Source: CAD feature listing. Evaluate the final solid. Frame: model axes, mm. A direction names the side the tool comes from. Coordinates: 2 decimals unless noted, no trailing zeros. Write each loop counter-clockwise with the first axis right and the second up, starting at its lowest first coordinate (ties: lowest second). Pieces come first, ordered by that corner, then holes. Notation, with made-up numbers: (-11.75, 64.5) - (34.25, 64.5) arc R10 cw to (34.25, 73.5) - close; hole circle Ø6 at (77.5, 89.5). An arc over 180 degrees is marked (long way). One line per item, written item: value.
from build123d import *

# Parameters (mm, degrees)
SALIENTE_EXTRUIR1_DEPTH = 2
CROQUIS2_W              = 12.25
CROQUIS2_H              = 10
SALIENTE_EXTRUIR2_DEPTH = 7
REDONDEO1_R             = 5
CROQUIS3_R              = 0.6
CORTAR_EXTRUIR1_DEPTH   = 7.2
SALIENTE_EXTRUIR3_DEPTH = 1.8
CROQUIS5_W              = 12.25
CROQUIS5_H              = 15.8
SALIENTE_EXTRUIR4_DEPTH = 7
REDONDEO2_R             = 5
CROQUIS6_R              = 0.6
CORTAR_EXTRUIR2_DEPTH   = 9.8
CROQUIS7_W              = 2.8
CROQUIS7_H              = 5.8
SALIENTE_EXTRUIR5_DEPTH = 1.8
CROQUIS8_R              = 1.5
CORTAR_EXTRUIR3_DEPTH   = 13.8
CROQUIS9_R              = 3
CORTAR_EXTRUIR4_DEPTH   = 6
CROQUIS10_R             = 12
SALIENTE_EXTRUIR6_DEPTH = 2
CORTAR_EXTRUIR5_DEPTH   = 2.2
CROQUIS12_R             = 1.6
CORTAR_EXTRUIR6_DEPTH   = 4.2
CROQUIS14_R             = 1.6
SALIENTE_EXTRUIR7_DEPTH = 2


with BuildPart() as part:
    # Croquis1 → Saliente-Extruir1 (new body)
    with BuildSketch(Plane(origin=(0, 0, 45.55), x_dir=(-1, 0, 0), z_dir=(0, 0, -1))):
        with BuildLine():
            Line((-17.240678969, 0.142768675), (-17.240678969, -9.857231325))
            ThreePointArc((-17.240678969, -9.857231325), (-7.189890991, -10.796826624), (2.512589694, -13.583051105))
            ThreePointArc((2.512589694, -13.583051105), (7.914003263, -15.134154499), (13.509321031, -15.657231325))
            Line((13.509321031, -15.657231325), (25.509321031, -15.657231325))
            Line((25.509321031, -15.657231325), (25.509321031, -3.657231325))
            ThreePointArc((25.509321031, -3.657231325), (21.994602405, 4.82805005), (13.509321031, 8.342768675))
            ThreePointArc((13.509321031, 8.342768675), (1.641917085, 6.787620461), (-9.424079639, 2.227195163))
            ThreePointArc((-9.424079639, 2.227195163), (-13.195803851, 0.672823972), (-17.240678969, 0.142768675))
        make_face()
    extrude(amount=SALIENTE_EXTRUIR1_DEPTH)

    # Croquis2 → Saliente-Extruir2 (add)
    with BuildSketch(Plane(origin=(17.240678969, 0, 0), x_dir=(0, 0, -1), z_dir=(1, 0, 0))):
        with Locations((-49.675, -4.857231325)):
            Rectangle(CROQUIS2_W, CROQUIS2_H)
    extrude(amount=SALIENTE_EXTRUIR2_DEPTH)

    # Redondeo1
    redondeo1_edges = [part.edges().sort_by_distance(p)[0] for p in [
        (24.240678969, -9.857231325, 49.675),
    ]]
    fillet(redondeo1_edges, radius=REDONDEO1_R)

    # Croquis3 → Cortar-Extruir1 (cut)
    with BuildSketch(Plane(origin=(0, 0.142768675, 0), x_dir=(1, 0, 0), z_dir=(0, 1, 0))):
        with Locations(Location((20.740678969, -50.8, 0), (0, 0, 270))):
            Circle(CROQUIS3_R)
    extrude(amount=-CORTAR_EXTRUIR1_DEPTH, mode=Mode.SUBTRACT)

    # Croquis4 → Saliente-Extruir3 (add)
    with BuildSketch(Plane.XY.offset(55.8)):
        with BuildLine():
            Line((19.340678969, -1.957231325), (19.340678969, -7.755506674))
            ThreePointArc((19.340678969, -7.755506674), (21.32634433, -6.872175493), (22.140678969, -4.857231325))
            Line((22.140678969, -4.857231325), (22.140678969, -1.957231325))
            Line((22.140678969, -1.957231325), (19.340678969, -1.957231325))
        make_face()
    extrude(amount=SALIENTE_EXTRUIR3_DEPTH)

    # Croquis5 → Saliente-Extruir4 (add)
    with BuildSketch(Plane.ZY.offset(23.759321031)):
        with Locations((49.675, -7.757231325)):
            Rectangle(CROQUIS5_W, CROQUIS5_H)
    extrude(amount=SALIENTE_EXTRUIR4_DEPTH)

    # Redondeo2
    redondeo2_edges = [part.edges().sort_by_distance(p)[0] for p in [
        (-30.759321031, -15.657231325, 49.675),
    ]]
    fillet(redondeo2_edges, radius=REDONDEO2_R)

    # Croquis6 → Cortar-Extruir2 (cut)
    with BuildSketch(Plane(origin=(0, 0.142768675, 0), x_dir=(1, 0, 0), z_dir=(0, 1, 0))):
        with Locations(Location((-27.259321031, -50.8, 0), (0, 0, 270))):
            Circle(CROQUIS6_R)
    extrude(amount=-CORTAR_EXTRUIR2_DEPTH, mode=Mode.SUBTRACT)

    # Croquis7 → Saliente-Extruir5 (add)
    with BuildSketch(Plane.XY.offset(55.8)):
        with Locations((-27.259321031, -4.857231325)):
            Rectangle(CROQUIS7_W, CROQUIS7_H)
    extrude(amount=SALIENTE_EXTRUIR5_DEPTH)

    # Croquis8 → Cortar-Extruir3 (cut)
    with BuildSketch(Plane.XY.offset(55.8)):
        with Locations((-27.259321031, -10.857231325)):
            Circle(CROQUIS8_R)
    extrude(amount=-CORTAR_EXTRUIR3_DEPTH, mode=Mode.SUBTRACT)

    # Croquis9 → Cortar-Extruir4 (cut)
    with BuildSketch(Plane(origin=(0, 0, 43.55), x_dir=(-1, 0, 0), z_dir=(0, 0, -1))):
        with Locations((27.259321031, -10.857231325)):
            Circle(CROQUIS9_R)
    extrude(amount=-CORTAR_EXTRUIR4_DEPTH, mode=Mode.SUBTRACT)

    # Croquis10 → Saliente-Extruir6 (add)
    with BuildSketch(Plane(origin=(0, 0, 43.55), x_dir=(-1, 0, 0), z_dir=(0, 0, -1))):
        with Locations(Location((13.509321031, -3.657231325, 0), (0, 0, 90))):
            Circle(CROQUIS10_R)
    extrude(amount=SALIENTE_EXTRUIR6_DEPTH)

    # Croquis11 → Cortar-Extruir5 (cut)
    with BuildSketch(Plane.XY.offset(45.55)):
        Polygon((-15.097034272, -0.907231325), (-16.684747512, -3.657231325), (-15.097034272, -6.407231325), (-11.921607791, -6.407231325), (-10.333894551, -3.657231325), (-11.921607791, -0.907231325), align=None)
    extrude(amount=-CORTAR_EXTRUIR5_DEPTH, mode=Mode.SUBTRACT)

    # Croquis12 → Cortar-Extruir6 (cut)
    with BuildSketch(Plane.XY.offset(45.55)):
        with Locations((-13.509321031, -3.657231325)):
            Circle(CROQUIS12_R)
    extrude(amount=-CORTAR_EXTRUIR6_DEPTH, mode=Mode.SUBTRACT)

    # Croquis14 → Saliente-Extruir7 (add)
    with BuildSketch(Plane(origin=(0, 0, 41.55), x_dir=(-1, 0, 0), z_dir=(0, 0, -1))):
        Polygon((13.509321031, 0.961570829), (9.509321031, -1.347830248), (9.509321031, -5.966632401), (13.509321031, -8.276033478), (17.509321031, -5.966632401), (17.509321031, -1.347830248), align=None)
        with Locations(Location((13.509321031, -3.657231325, 0), (0, 0, 180))):
            Circle(CROQUIS14_R, mode=Mode.SUBTRACT)
    extrude(amount=SALIENTE_EXTRUIR7_DEPTH)


solid = part.part
1) Contact query for flat-ended pins moving along their axis: P1, Ø0.5, axis at y = -4.5, z = 57, coming from the -X side; P2, Ø2, axis at x = 18.5, z = 50.5, coming from the -Y side; P3, Ø8, axis at x = -23.5, z = 51, coming from the +Y side. Output: stop coordinate, or through.
Values found:
P1: x = -28.66
P2: y = -9.86
P3: y = 0.14
2) Section query D-D on x = -7. Output: boundary loops of the cut face in (y, z).
Values found:
outline: (-14.95, 43.55) - (-13.74, 43.55) - (-13.74, 41.55) - (6.42, 41.55) - (6.42, 43.55) - (7.88, 43.55) - (7.88, 45.55) - (-14.95, 45.55) - close
3) Material intervals for line 1 (X direction, y = -4, z = 50.8); line 2 (X direction, y = -8.5, z = 47.5); line 3 (X direction, y = -9.25, z = 47.5), sorted ascending.
Values found:
line 1: -30.76 to -27.86, -26.66 to -23.76, 17.24 to 20.14, 21.34 to 24.24
line 2: -30.76 to -29.11, -25.4 to -23.76, 17.24 to 22.67
line 3: -30.76 to -29.79, -24.73 to -23.76, 17.24 to 21.63
4) Section query A-A on z = 54.5. Output: boundary loops of the cut face in (x, y).
Values found:
outline: (-30.76, -10.66) arc R5 ccw to (-25.76, -15.66) - (-23.76, -15.66) - (-23.76, 0.14) - (-30.76, 0.14) - close; (17.24, -9.86) - (19.24, -9.86) arc R5 ccw to (24.24, -4.86) - (24.24, 0.14) - (17.24, 0.14) - close; hole circle Ø3 at (-27.26, -10.86)
5) Draft query along X for faces 1 (the flat face through (-28.659, -5, 57)), 2 (the cylindrical face through (22.74, -8.43, 49.59)), 3 (the flat face through (-11.14, -5.05, 44.47)), 4 (the flat face through (-27, -1.957, 57)). Return one class per face: released by +X, released by -X, zero draft, split by the parting line, or undercut.
Values found:
face 1: released by -X
face 2: released by +X
face 3: undercut
face 4: zero draft
6) Section query B-B on z = 50.8. Output: boundary loops of the cut face in (x, y), then the cut area to 3 significant figures.
Values found:
outline: (-30.76, -10.66) arc R5 ccw to (-25.76, -15.66) - (-23.76, -15.66) - (-23.76, 0.14) - (-26.66, 0.14) - (-26.66, -9.48) arc R1.5 cw (long way) to (-27.86, -9.48) - (-27.86, 0.14) - (-30.76, 0.14) - close; (17.24, -9.86) - (19.24, -9.86) arc R5 ccw to (24.24, -4.86) - (24.24, 0.14) - (21.34, 0.14) - (21.34, -7.06) - (20.14, -7.06) - (20.14, 0.14) - (17.24, 0.14) - close
area: 143 mm2
7) Reachability of faces 5 (the flat face through (-15.54, -0.21, 40.56)), 6 (the flat face through (-27, 0.143, 50)), 7 (the flat face through (-11.5, -0.2, 40.6)), 8 (the flat face through (22.141, -3, 57)), 9 (the flat face through (-28, -9, 49.55)) from +Z, -Z, +X, -X, +Y, -Y: full face, straight path, thin tool, end or side. Return the list, or none.
Values found:
face 5: -Z, -X, +Y
face 6: +Z, -X, +Y
face 7: -Z, +X, +Y
face 8: +Z, +X, +Y, -Y
face 9: -Z
8) Section query C-C on y = 6.25. Output: boundary loops of the cut face in (x, z).
Values found:
outline: (-20.28, 41.55) - (-6.74, 41.55) - (-6.74, 43.55) - (0.22, 43.55) - (0.22, 45.55) - (-20.28, 45.55) - close
